from build123d import *

# Parameters (mm, degrees)
SKETCH1_W           = 101.6
SKETCH1_H           = 57.15
BOSS_EXTRUDE1_DEPTH = 3.175
SKETCH2_W           = 12.7
SKETCH2_H           = 6.35
CUT_EXTRUDE1_DEPTH  = 59.630138368


with BuildPart() as part:
    # Sketch1 → Boss-Extrude1 (new, symmetric)
    with BuildSketch(Plane.XY):
        Rectangle(SKETCH1_W, SKETCH1_H)
    extrude(amount=BOSS_EXTRUDE1_DEPTH, both=True)

    # Sketch2 → Cut-Extrude1 (cut, through all)
    with BuildSketch(Plane.XY.offset(3.175)):
        with Locations((-44.45, 25.4)):
            Rectangle(SKETCH2_W, SKETCH2_H)
    cut_extrude1 = extrude(amount=-CUT_EXTRUDE1_DEPTH, mode=Mode.SUBTRACT)

    # Mirror1: Cut-Extrude1 across plane
    add(cut_extrude1.mirror(Plane(origin=(0, 0, 0), x_dir=(0, 0, 1), z_dir=(1, 0, 0))), mode=Mode.SUBTRACT)


solid = part.part
Work out the finished part from the listing and answer in its coordinate system (mm). A direction names the side the tool comes from. Give positions to 0.01 mm unless a question says otherwise; leave off trailing zeros. Order: outer loops, then holes, each group sorted by start corner. A loop starts at its lowest first (then second) coordinate and runs counter-clockwise, first axis right, second up. Notation, with made-up numbers: (16.5, 65) -> (32.5, 65) arc R21 cw to (32.5, 94) -> close; hole circle Ø8 at (9, 18.5). An arc over 180 degrees is marked (long way). Answer as a JSON object with one key per item and string values. Group by question number.
1. A tool of negligible diameter and unlimited length cuts with its end or side. For faces 1 (the flat face through (38.1, 25, 0)), 2 (the flat face through (-38.1, 25, 0)), 3 (the flat face through (-50.8, -4, 0)), from which of +Z, -Z, +X, -X, +Y, -Y can it reach the whole face along a straight path? Write none if from no direction.
2. Section B-B on x = -42.5 is taken. Determine the outline of the cut face in (y, z) (3 decimals).
3. Consider line 1 along Y through (x, z) = (39, 2.5) (3 decimals); line 2 along X through (y, z) = (26, 0.25). Determine where each line is inside the solid, lowest interval first. Write a range as [from, to].
4. Flat-ended cylindrical pins translate along their axes: pin 1 Ø1.9 at (y, z) = (25, 0) entering from +X; pin 2 Ø1.9 at (x, z) = (-42, -0.5) entering from +Y (3 decimals). Find the tip coordinate at first contact, or state that the pin passes through.
5. Section A-A on z = -1.5 is taken. Determine the outline of the cut face in (x, y) (3 decimals), plus the area to 3 significant figures.
Result sheet:
{
 "1": {"face 1": "+Z, -Z, +X, +Y", "face 2": "+Z, -Z, -X, +Y", "face 3": "+Z, -Z, -X, +Y, -Y"},
 "2": {"outline": "(-28.575, -3.175) -> (22.225, -3.175) -> (22.225, 3.175) -> (-28.575, 3.175) -> close"},
 "3": {"line 1": "y = [-28.575, 22.225]", "line 2": "x = [-38.1, 38.1]"},
 "4": {"pin 1": "stops at x = 38.1", "pin 2": "stops at y = 22.225"},
 "5": {"outline": "(-50.8, -28.575) -> (50.8, -28.575) -> (50.8, 22.225) -> (38.1, 22.225) -> (38.1, 28.575) -> (-38.1, 28.575) -> (-38.1, 22.225) -> (-50.8, 22.225) -> close", "area": "5,650 mm^2"}
}
